```python
from build123d import *

# Parameters (mm, degrees)
EXTRUDE_1_DEPTH = 1
EXTRUDE_2_DEPTH = 0.5


with BuildPart() as part:
    # 草图1 → 凸台-拉伸1 (new body)
    with BuildSketch(Plane(origin=(0, 0, 0), x_dir=(1, 0, 0), z_dir=(0, 1, 0))):
        Polygon((-31.25, 0), (31.25, 0), (21.75, 73.5), (-21.75, 73.5), align=None)
    extrude(amount=EXTRUDE_1_DEPTH)

    # 草图2 → 凸台-拉伸2 (add)
    with BuildSketch(Plane(origin=(0, 1, 0), x_dir=(1, 0, 0), z_dir=(0, 1, 0))):
        Polygon((-21.75, 73.5), (-31.25, 0), (31.25, 0), (21.75, 73.5), align=None)
        Polygon((-20.870933298, 72.5), (-30.112429896, 1), (30.112429896, 1), (20.870933298, 72.5), align=None, mode=Mode.SUBTRACT)
    extrude(amount=EXTRUDE_2_DEPTH)


solid = part.part
```
Verification items for the finished model (mm, model axes). A direction names the side the tool comes from. Coordinates: 2 decimals unless noted, no trailing zeros. Loops run counter-clockwise (first coordinate to the right, second up) from the corner with the lowest first, then second, coordinate; pieces in that order, holes last. Notation, with made-up numbers: (66.25, 11) - (93.25, 11) arc R13 cw to (93.25, 21) - close; hole circle Ø8 at (84, 2.25). An arc over 180 degrees is marked (long way). Return JSON: item names as keys, results as strings.
1. Section check C-C, the plane y = 0.4. Record the boundary of the cut face in (x, z).
Established:
{"outline": "(-31.25, 0) - (-21.75, -73.5) - (21.75, -73.5) - (31.25, 0) - close"}
2. Mould release check, pull along X, two halves, no side actions. Record for faces 3 (the flat face through (25.556, 1.246, -36.25)), 4 (the flat face through (0, 1, -73.5)), 5 (the flat face through (-26.434, 0.74, -37.264)), 6 (the flat face through (26.566, 0.74, -36.236)): +X half, -X half, draft (parallel to the pull), parting line (faces both ways), or undercut.
Established:
{"face 3": "undercut", "face 4": "draft", "face 5": "-X half", "face 6": "+X half"}
3. Go/stop test with flat-tipped pins: pin 1 (4 mm diameter, centred on x = 10, z = -44, fed in from +Y); pin 2 (1 mm diameter, centred on x = -14.5, z = -43, fed in from -Y). Record where each tip stops, or that it passes through.
Established:
{"pin 1": "stops at y = 1", "pin 2": "stops at y = 0"}
4. Thickness scan on L1, parallel to Z at x = 1.5, y = 1.25; L2, parallel to Y at x = -14, z = -45.5; L3, parallel to X at y = 1.3, z = -48. Record the ranges inside material, lowest first.
Established:
{"L1": "z = -73.5 to -72.5, -1 to 0", "L2": "y = 0 to 1", "L3": "x = -25.05 to -24.04, 24.04 to 25.05"}
5. Tool access check on faces 1 (the flat face through (-26, 1.5, -37)), 2 (the flat face through (0, 1, -37)). Record the directions out of +Z, -Z, +X, -X, +Y, -Y that give a thin tool (end or side, any length) a straight path to the whole face; none if there is none.
Established:
{"face 1": "+Z, -Z, +X, -X, +Y", "face 2": "+Y"}
6. Section check B-B, the plane z = -46.5. Record the boundary of the cut face in (x, y), then the cut area to 3 significant figures.
Established:
{"outline": "(-25.24, 0) - (25.24, 0) - (25.24, 1.5) - (24.23, 1.5) - (24.23, 1) - (-24.23, 1) - (-24.23, 1.5) - (-25.24, 1.5) - close", "area": "51.5 mm2"}
7. Section check A-A, the plane x = -4.5. Record the boundary of the cut face in (y, z), then the cut area to 3 significant figures.
Established:
{"outline": "(0, -73.5) - (1.5, -73.5) - (1.5, -72.5) - (1, -72.5) - (1, -1) - (1.5, -1) - (1.5, 0) - (0, 0) - close", "area": "74.5 mm2"}
